from build123d import *

# Parameters (mm, degrees)
SKETCH1_W           = 40
SKETCH1_H           = 70
BOSS_EXTRUDE1_DEPTH = 3
BOSS_EXTRUDE2_DEPTH = 20
BOSS_EXTRUDE3_DEPTH = 20
CUT_EXTRUDE1_DEPTH  = 13
BOSS_EXTRUDE4_DEPTH = 10
FILLET1_R           = 5
CUT_EXTRUDE2_REACH  = 43.533
SKETCH5_R           = 2.75
CUT_EXTRUDE4_DEPTH  = 2


with BuildPart() as part:
    # Sketch1 → Boss-Extrude1 (new body)
    with BuildSketch(Plane.XY):
        Rectangle(SKETCH1_W, SKETCH1_H)
    extrude(amount=BOSS_EXTRUDE1_DEPTH)

    # Sketch2 → Boss-Extrude2 (add, symmetric)
    with BuildSketch(Plane(origin=(0, 0, 0), x_dir=(0, 0, -1), z_dir=(1, 0, 0))):
        Polygon((0, 29), (10, 29), (10, 23), (7.154700538, 23), (6, 25), (5, 25), (5, 21), (0, 21), align=None)
    extrude(amount=BOSS_EXTRUDE2_DEPTH, both=True)

    # Sketch3 → Boss-Extrude3 (add, symmetric)
    with BuildSketch(Plane(origin=(0, 0, 0), x_dir=(0, 0, -1), z_dir=(1, 0, 0))):
        Polygon((0, -18), (10, -18), (10, -9), (7.057961884, -9), (6, -15), (5, -15), (5, -2), (0, -2), align=None)
    extrude(amount=BOSS_EXTRUDE3_DEPTH, both=True)

    # Sketch3_2 → Cut-Extrude1 (cut, symmetric)
    with BuildSketch(Plane(origin=(0, 0, 0), x_dir=(0, 0, -1), z_dir=(1, 0, 0))):
        Polygon((0, -18), (10, -18), (10, -9), (7.057961884, -9), (6, -15), (5, -15), (5, -2), (0, -2), align=None)
    extrude(amount=CUT_EXTRUDE1_DEPTH, both=True, mode=Mode.SUBTRACT)

    # Sketch4 → Boss-Extrude4 (add)
    with BuildSketch(Plane.XY):
        with BuildLine():
            Line((13, -18), (-13, -18))
            Line((-13, -18), (-13, -15))
            Line((-13, -15), (11.2, -15))
            add(Edge.make_bspline(
                [(11.2, -15), (7.988659261, -12.305365171), (4.131076897, -9.981226783), (-4.059161179, -9.974707843), (-6.438372816, -13.757567443), (-9.210423341, -14.299843052), (-11, -12.5)],
                knots=[0, 0, 0, 0, 0.361861055, 0.44515142, 0.789820069, 1, 1, 1, 1], degree=3))
            Line((-11, -12.5), (-11, -11.5))
            add(Edge.make_bspline(
                [(13, -15), (9.091847393, -11.720670589), (5.160163517, -9.012654879), (-4.52853577, -8.942546967), (-6.581487755, -13.325064148), (-9.8688482, -13.174994697), (-11, -11.5)],
                knots=[0, 0, 0, 0, 0.360137541, 0.439165428, 0.751266273, 1, 1, 1, 1], degree=3))
            Line((13, -15), (13, -18))
        make_face()
    extrude(amount=-BOSS_EXTRUDE4_DEPTH)

    # Fillet1
    fillet1_edges = [part.edges().sort_by_distance(p)[0] for p in [
        (20, -35, 1.5),
        (-20, -35, 1.5),
        (-20, 35, 1.5),
        (20, 35, 1.5),
    ]]
    fillet(fillet1_edges, radius=FILLET1_R)

    # Sketch5 → Cut-Extrude2 (cut, up to next)
    with BuildSketch(Plane.XY, mode=Mode.PRIVATE) as cut_extrude2_sk1:
        with Locations(Location((-12, 16, 0), (0, 0, 180))):
            Circle(SKETCH5_R)
    cut_extrude2_tool1 = extrude(cut_extrude2_sk1.sketch, amount=CUT_EXTRUDE2_REACH, mode=Mode.PRIVATE) & part.part
    # Sketch5 → Cut-Extrude2 (cut, up to next)
    with BuildSketch(Plane.XY, mode=Mode.PRIVATE) as cut_extrude2_sk2:
        with Locations(Location((12, 16, 0), (0, 0, 180))):
            Circle(SKETCH5_R)
    cut_extrude2_tool2 = extrude(cut_extrude2_sk2.sketch, amount=CUT_EXTRUDE2_REACH, mode=Mode.PRIVATE) & part.part
    # Sketch5 → Cut-Extrude2 (cut, up to next)
    with BuildSketch(Plane.XY, mode=Mode.PRIVATE) as cut_extrude2_sk3:
        with Locations(Location((-12, -24, 0), (0, 0, 180))):
            Circle(SKETCH5_R)
    cut_extrude2_tool3 = extrude(cut_extrude2_sk3.sketch, amount=CUT_EXTRUDE2_REACH, mode=Mode.PRIVATE) & part.part
    # Sketch5 → Cut-Extrude2 (cut, up to next)
    with BuildSketch(Plane.XY, mode=Mode.PRIVATE) as cut_extrude2_sk4:
        with Locations(Location((12, -24, 0), (0, 0, 180))):
            Circle(SKETCH5_R)
    cut_extrude2_tool4 = extrude(cut_extrude2_sk4.sketch, amount=CUT_EXTRUDE2_REACH, mode=Mode.PRIVATE) & part.part
    add(cut_extrude2_tool1.solids().sort_by_distance((-12, 16, 0))[0], mode=Mode.SUBTRACT)
    add(cut_extrude2_tool2.solids().sort_by_distance((12, 16, 0))[0], mode=Mode.SUBTRACT)
    add(cut_extrude2_tool3.solids().sort_by_distance((-12, -24, 0))[0], mode=Mode.SUBTRACT)
    add(cut_extrude2_tool4.solids().sort_by_distance((12, -24, 0))[0], mode=Mode.SUBTRACT)

    # Sketch4_2 → Cut-Extrude4 (cut)
    with BuildSketch(Plane.XY):
        with BuildLine():
            Line((13, -18), (-13, -18))
            Line((-13, -18), (-13, -15))
            Line((-13, -15), (11.2, -15))
            add(Edge.make_bspline(
                [(11.2, -15), (7.988659261, -12.305365171), (4.131076897, -9.981226783), (-4.059161179, -9.974707843), (-6.438372816, -13.757567443), (-9.210423341, -14.299843052), (-11, -12.5)],
                knots=[0, 0, 0, 0, 0.361861055, 0.44515142, 0.789820069, 1, 1, 1, 1], degree=3))
            Line((-11, -12.5), (-11, -11.5))
            add(Edge.make_bspline(
                [(13, -15), (9.091847393, -11.720670589), (5.160163517, -9.012654879), (-4.52853577, -8.942546967), (-6.581487755, -13.325064148), (-9.8688482, -13.174994697), (-11, -11.5)],
                knots=[0, 0, 0, 0, 0.360137541, 0.439165428, 0.751266273, 1, 1, 1, 1], degree=3))
            Line((13, -15), (13, -18))
        make_face()
    extrude(amount=-CUT_EXTRUDE4_DEPTH, mode=Mode.SUBTRACT)


solid = part.part
Geometry check sheet. Reference: the model listing, model coordinates, mm. A direction names the side the tool comes from. Coordinates: 2 decimals unless noted, no trailing zeros. Order: outer loops, then holes, each group sorted by start corner. A loop starts at its lowest first (then second) coordinate and runs counter-clockwise, first axis right, second up. Notation, with made-up numbers: (43.5, 25) - (58.5, 25) arc R7 cw to (58.5, 34) - close; hole circle Ø11 at (49.5, 77.25). An arc over 180 degrees is marked (long way). Answer in a Markdown table with one row per item. Add a question column.
1) Cross-section at A-A, the plane y = 16. Record the cut outline in (x, z), then the cut area to 3 significant figures.
2) Cross-section at B-B, the plane x = -12. Record the cut outline in (y, z).
3) Gauge pin test, flat ends, axial feed: P1, Ø5.5, axis at x = 1, z = -3.5, coming from the -Y side; P2, Ø1.5, axis at x = 15.5, z = -8, coming from the +Y side; P3, Ø7, axis at x = -12, y = -24, coming from the -Z side; P4, Ø2, axis at y = 4.5, z = -2, coming from the +X side. Record the tip position at first contact, or that the pin passes through.
4) Cross-section at C-C, the plane z = 1.5. Record the cut outline in (x, y).
5) Cross-section at D-D, the plane y = -20. Record the cut outline in (x, z), then the cut area to 3 significant figures.
6) Set-up check for faces 1 (the cylindrical face through (-19, 33, 2)), 2 (the flat face through (17, -2, -3)), 3 (the flat face through (-13, -12, -8)): record each of +Z, -Z, +X, -X, +Y, -Y from which the full face is reachable in a straight line by a thin tool's end or side.
7) Material ranges on line 1 along Y through (x, z) = (12, 1.1); line 2 along X through (y, z) = (-24, 2.1); line 3 along Y through (x, z) = (18.5, -5.25), recorded low to high. Write a range as [from, to].
8) Release check for a two-part mould opening along Z. For faces 4 (the flat face through (-16.451, -11.958, -6.536)), 5 (the flat face through (16.549, -11.958, -6.536)), 6 (the flat face through (0, 0, 3)), 7 (the cylindrical face through (-11.642, 13.273, 1.479)) record: +Z half, -Z half, draft (parallel to the pull), parting line (faces both ways), or undercut.
Check result:
| question | item | result |
|---|---|---|
| 1 | outline | (-20, 0) - (-14.75, 0) - (-14.75, 3) - (-20, 3) - close; (-9.25, 0) - (9.25, 0) - (9.25, 3) - (-9.25, 3) - close; (14.75, 0) - (20, 0) - (20, 3) - (14.75, 3) - close |
| 1 | area | 87.0 mm² |
| 2 | outline | (-35, 0) - (-26.75, 0) - (-26.75, 3) - (-35, 3) - close; (-21.25, 0) - (13.25, 0) - (13.25, 3) - (-21.25, 3) - close; (-18, -10) - (-15, -10) - (-15, -2) - (-18, -2) - close; (18.75, 0) - (21, 0) - (21, -5) - (25, -5) - (25, -6) - (23, -7.15) - (23, -10) - (29, -10) - (29, 0) - (35, 0) - (35, 3) - (18.75, 3) - close |
| 3 | P1 | stops at y = -18 |
| 3 | P2 | stops at y = 29 |
| 3 | P3 | stops at z = 0 |
| 3 | P4 | passes through |
| 4 | outline | (-20, -30) arc R5 ccw to (-15, -35) - (15, -35) arc R5 ccw to (20, -30) - (20, 30) arc R5 ccw to (15, 35) - (-15, 35) arc R5 ccw to (-20, 30) - close; hole circle Ø5.5 at (-12, -24); hole circle Ø5.5 at (-12, 16); hole circle Ø5.5 at (12, -24); hole circle Ø5.5 at (12, 16) |
| 5 | outline | (-20, 0) - (20, 0) - (20, 3) - (-20, 3) - close |
| 5 | area | 120 mm² |
| 6 | face 1 | +Z, -Z, -X, +Y |
| 6 | face 2 | -Z, +X, -X |
| 6 | face 3 | -Z |
| 7 | line 1 | y = [-35, -26.75], [-21.25, 13.25], [18.75, 35] |
| 7 | line 2 | x = [-20, -14.75], [-9.25, 9.25], [14.75, 20] |
| 7 | line 3 | y = [-18, -15], [25, 29] |
| 8 | face 4 | undercut |
| 8 | face 5 | undercut |
| 8 | face 6 | +Z half |
| 8 | face 7 | draft |
